```python
from build123d import *

# Parameters (mm, degrees)
F0_W      = 137.3124
F0_H      = 89.6874
F1_DEPTH  = 3.175
F3_R      = 3.81
F4_DEPTH  = 19.05
F5_W      = 137.3124
F5_H      = 89.6874
F6_DEPTH  = 3.175
F2_R      = 6.35
F8_DEPTH  = 6.35
F7_R      = 4.365625
F9_DEPTH  = 25.4
F10_R     = 4.306197
F10_R_2   = 4.1275
F11_DEPTH = 6.35


with BuildPart() as f1:
    # F0 (on Top) → F1 (new body)
    with BuildSketch(Plane.XY):
        with Locations((3.890783, 13.083767)):
            Rectangle(F0_W, F0_H)
    extrude(amount=-F1_DEPTH)

    # F3 (on face) → F4 (join)
    with BuildSketch(Plane(origin=(0, 0, -3.175), x_dir=(1, 0, 0), z_dir=(0, 0, -1))):
        with Locations((-57.145417, 24.139933)):
            Circle(F3_R)
        with Locations((64.926983, 24.139933)):
            Circle(F3_R)
        with Locations((-57.145417, -50.307467)):
            Circle(F3_R)
        with Locations((64.926983, -50.307467)):
            Circle(F3_R)
        with Locations((-8.606017, -13.083767)):
            Circle(F3_R)
        with Locations((16.387583, -13.083767)):
            Circle(F3_R)
    extrude(amount=F4_DEPTH)

    # F5 (on face) → F6 (join)
    with BuildSketch(Plane(origin=(0, 0, -22.225), x_dir=(1, 0, 0), z_dir=(0, 0, -1))):
        with Locations((3.875781, -12.945777)):
            Rectangle(F5_W, F5_H)
    extrude(amount=F6_DEPTH)

    # F2 (on face) → F8 (cut)
    with BuildSketch(Plane.XY):
        with Locations((-46.121817, 43.799987)):
            Circle(F2_R)
        with Locations((-21.128217, 43.799987)):
            Circle(F2_R)
        with Locations((3.865383, 43.799987)):
            Circle(F2_R)
        with Locations((28.858983, 43.799987)):
            Circle(F2_R)
        with Locations((53.852583, 43.799987)):
            Circle(F2_R)
        with Locations((-46.121817, -17.632453)):
            Circle(F2_R)
        with Locations((-21.128217, -17.632453)):
            Circle(F2_R)
        with Locations((3.865383, -17.632453)):
            Circle(F2_R)
        with Locations((28.858983, -17.632453)):
            Circle(F2_R)
        with Locations((53.852583, -17.632453)):
            Circle(F2_R)
        with Locations((-46.121817, 23.322507)):
            Circle(F2_R)
        with Locations((-21.128217, 23.322507)):
            Circle(F2_R)
        with Locations((3.865383, 23.322507)):
            Circle(F2_R)
        with Locations((28.858983, 23.322507)):
            Circle(F2_R)
        with Locations((53.852583, 23.322507)):
            Circle(F2_R)
        with Locations((-46.121817, 2.845027)):
            Circle(F2_R)
        with Locations((-21.128217, 2.845027)):
            Circle(F2_R)
        with Locations((3.865383, 2.845027)):
            Circle(F2_R)
        with Locations((28.858983, 2.845027)):
            Circle(F2_R)
        with Locations((53.852583, 2.845027)):
            Circle(F2_R)
    extrude(amount=-F8_DEPTH, mode=Mode.SUBTRACT)

    # F7 (on face) → F9 (cut)
    with BuildSketch(Plane(origin=(0, 0, -25.4), x_dir=(1, 0, 0), z_dir=(0, 0, -1))):
        with Locations((-46.136819, 17.770443)):
            Circle(F7_R)
        with Locations((-21.143219, 17.770443)):
            Circle(F7_R)
        with Locations((3.850381, 17.770443)):
            Circle(F7_R)
        with Locations((28.843981, 17.770443)):
            Circle(F7_R)
        with Locations((53.837581, 17.770443)):
            Circle(F7_R)
        with Locations((-46.136819, -2.707037)):
            Circle(F7_R)
        with Locations((-21.143219, -2.707037)):
            Circle(F7_R)
        with Locations((3.850381, -2.707037)):
            Circle(F7_R)
        with Locations((28.843981, -2.707037)):
            Circle(F7_R)
        with Locations((53.837581, -2.707037)):
            Circle(F7_R)
        with Locations((-46.136819, -23.184517)):
            Circle(F7_R)
        with Locations((-21.143219, -23.184517)):
            Circle(F7_R)
        with Locations((3.850381, -23.184517)):
            Circle(F7_R)
        with Locations((28.843981, -23.184517)):
            Circle(F7_R)
        with Locations((53.837581, -23.184517)):
            Circle(F7_R)
        with Locations((-46.136819, -43.661997)):
            Circle(F7_R)
        with Locations((-21.143219, -43.661997)):
            Circle(F7_R)
        with Locations((3.850381, -43.661997)):
            Circle(F7_R)
        with Locations((28.843981, -43.661997)):
            Circle(F7_R)
        with Locations((53.837581, -43.661997)):
            Circle(F7_R)
    extrude(amount=-F9_DEPTH, mode=Mode.SUBTRACT)

    # F10 (on face) → F11 (join)
    with BuildSketch(Plane(origin=(0, 0, -25.4), x_dir=(1, 0, 0), z_dir=(0, 0, -1))):
        with Locations((-57.160419, 24.277923)):
            Circle(F10_R)
        with Locations((64.911981, 24.277923)):
            Circle(F10_R_2)
        with Locations((64.911981, -50.169477)):
            Circle(F10_R_2)
        with Locations((-57.160419, -50.169477)):
            Circle(F10_R_2)
    extrude(amount=F11_DEPTH)


solid = f1.part
```
Can you work these out from the model? Positions are in its coordinate system, mm. A direction names the side the tool comes from. Coordinates: 2 decimals unless noted, no trailing zeros. Loops run counter-clockwise (first coordinate to the right, second up) from the corner with the lowest first, then second, coordinate; pieces in that order, holes last. Notation, with made-up numbers: M -12,5.25 L 33,5.25 A19 ccw 33,19.25 Z; hole C -31,77 d4. An arc over 180 degrees is marked long. Put each result on its own line as item: value. Start each with the question number.
(1) Which directions (+Z, -Z, +X, -X, +Y, -Y) give clear straight access to the entire face, cutting with the end or side of a thin tool? Please do faces 5 (the face through (6.8, 17.69, -1.57)), 6 (the face through (0.386, 5.363, -23.835)), 7 (the face through (3, 57.789, -24)).
(2) Imagine slicing it at D-D on z = -27. List the corners of the cut face in (x, y) for me (1 decimal).
(3) Imagine slicing it at B-B on z = -14. List the corners of the cut face in (x, y) for me.
(4) We'd pull the mould along Z, two halves only. Please class faces 1 (the face through (3, 14, -3.175)), 2 (the face through (3, 14, 0)), 3 (the face through (65, -24, -31.75)), 4 (the face through (-40.065, 45.707, -1.565)): +Z half, -Z half, draft (parallel to the pull), parting line (faces both ways), or undercut.
(5) Imagine slicing it at A-A on x = 44.5. List the corners of the cut face in (y, z) for me (3 decimals).
(6) I need wall thicknesses on probe 1 along Z at (x, y) = (59.5, -21) (3 decimals); probe 2 along Y at (x, z) = (-41, -2); probe 3 along Y at (x, z) = (41.5, -24.5). Which ranges of each line are inside material? Lowest first, please.
(7) Will these pins go through, and if not, where does the flat tip stop? pin 1 Ø11.5 at (x, y) = (28.84, 43.66) entering from -Z; pin 2 Ø7 at (x, y) = (-21.14, -17.77) entering from -Z; pin 3 Ø10 at (x, y) = (-21.14, 2.71) entering from +Z (3 decimals); pin 4 Ø5 at (y, z) = (21, -21.5) entering from +X.
(8) Imagine slicing it at C-C on y = 4.5. Give the number of separate pieces and of enclosed holes in the cut face, and give its area (3 significant figures).
Worked answers:
1. face 5: +Z
1. face 6: +Z, -Z
1. face 7: -Z, +X, -X, +Y
2. outline: C -57.2,-24.3 d8.6; C -57.2,50.2 d8.3; C 64.9,-24.3 d8.3; C 64.9,50.2 d8.3
3. outline: C -57.15,-24.14 d7.62; C -57.15,50.31 d7.62; C -8.61,13.08 d7.62; C 16.39,13.08 d7.62; C 64.93,-24.14 d7.62; C 64.93,50.31 d7.62
4. face 1: undercut
4. face 2: +Z half
4. face 3: -Z half
4. face 4: draft
5. outline: M -31.898,-25.4 L 57.789,-25.4 L 57.789,-22.225 L -31.898,-22.225 Z; M -31.76,-3.175 L 57.927,-3.175 L 57.927,0 L -31.76,0 Z
6. probe 1: z = -25.4 to -22.225, -3.175 to 0
6. probe 2: y = -31.76 to -21.39, -13.88 to -0.91, 6.6 to 19.57, 27.08 to 40.05, 47.55 to 57.93
6. probe 3: y = -31.9 to 57.79
7. pin 1: stops at z = -25.4
7. pin 2: passes through
7. pin 3: stops at z = -22.225
7. pin 4: stops at x = 72.53
8. separate pieces: 12
8. enclosed holes: 0
8. area: 551 mm2
